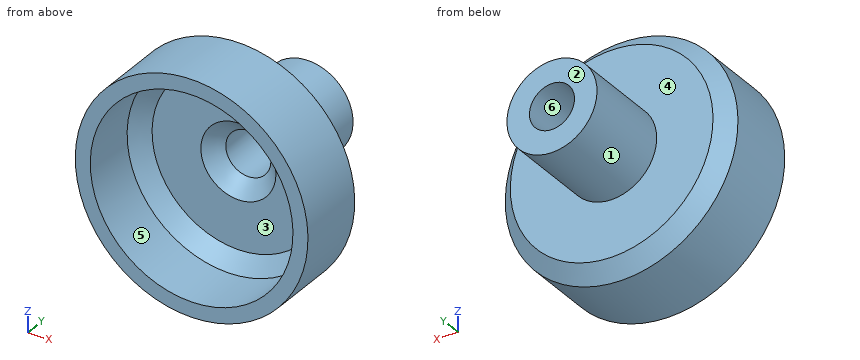
```python
from build123d import *

# Parameters (mm, degrees)
CHAMFER1_SIZE = 2
CHAMFER2_SIZE = 2


with BuildPart() as part:
    # Sketch1 → Revolve1 (revolve)
    with BuildSketch(Plane.XY, mode=Mode.PRIVATE) as revolve1_sk:
        Polygon((-15.5, 0), (-15.5, 11.4), (-6, 11.4), (-6, 23.4), (-3, 23.4), (-3, 9.4), (-13.5, 9.4), (-13.5, 0), align=None)
    revolve(revolve1_sk.sketch.rotate(Axis((0, 0, 0), (0, 1, 0)), 270), axis=Axis((0, 0, 0), (0, 1, 0)))

    # Chamfer1
    chamfer1_edges = [part.edges().sort_by_distance(p)[0] for p in [
        (0, 9.4, 13.5),
        (0, 11.4, 15.5),
    ]]
    chamfer(chamfer1_edges, length=CHAMFER1_SIZE)

    # Chamfer2
    chamfer2_edges = [part.edges().sort_by_distance(p)[0] for p in [
        (0, 9.4, 3),
    ]]
    chamfer(chamfer2_edges, length=CHAMFER2_SIZE)


solid = part.part
```
For this review, take the finished solid that the model builds, in its own axes (mm). Face numbers are marked on the shaded views. A direction names the side the tool comes from. Round coordinates to 2 decimals unless told otherwise and drop trailing zeros. Write each loop counter-clockwise with the first axis right and the second up, starting at its lowest first coordinate (ties: lowest second). Pieces come first, ordered by that corner, then holes.
1) Insertion check: pin 1 Ø1 at (x, y) = (4.5, 20) entering from +Z; pin 2 Ø1 at (y, z) = (6, 0.5) entering from -X; pin 3 Ø10 at (y, z) = (6.5, 8.5) entering from -X; pin 4 Ø1 at (x, z) = (-10, -7.5) entering from -Y. Each pin has a flat end and moves straight along its axis. Give the tip position at first contact, or say it passes through.
Answer below:
pin 1: stops at z = 4.47
pin 2: stops at x = -15.5
pin 3: stops at x = -15.1
pin 4: stops at y = 7.9
2) Take a section at A-A on x = 0. Give the boundary of the cut face in (y, z), then the cut area to 3 significant figures.
Answer below:
outline: (0, -15.5) - (9.4, -15.5) - (11.4, -13.5) - (11.4, -6) - (23.4, -6) - (23.4, -3) - (11.4, -3) - (9.4, -5) - (9.4, -11.5) - (7.4, -13.5) - (0, -13.5) - close; (0, 13.5) - (7.4, 13.5) - (9.4, 11.5) - (9.4, 5) - (11.4, 3) - (23.4, 3) - (23.4, 6) - (11.4, 6) - (11.4, 13.5) - (9.4, 15.5) - (0, 15.5) - close
area: 156 mm2
3) Mouldability with a two-part tool opening along Z and no side actions: class the marked faces 1, 2 and 3 as +Z half, -Z half, draft (parallel to the pull), parting line (faces both ways), or undercut.
Answer below:
face 1: parting line
face 2: draft
face 3: undercut
4) For line 1 along X through (y, z) = (14.5, 0); line 2 along X through (y, z) = (5.25, 0); line 3 along Y through (x, z) = (8.5, -6.5), list the stretches that pass through material, from the lowest coordinate up.
Answer below:
line 1: x = -6 to -3, 3 to 6
line 2: x = -15.5 to -13.5, 13.5 to 15.5
line 3: y = 9.4 to 11.4
5) Take a section at C-C on y = 15.5. Give the boundary of the cut face in (x, z).
Answer below:
outline: circle Ø12 at (0, 0); hole circle Ø6 at (0, 0)
6) Take a section at B-B on z = 0. Give the boundary of the cut face in (x, y).
Answer below:
outline: (-15.5, 0) - (-13.5, 0) - (-13.5, 7.4) - (-11.5, 9.4) - (-5, 9.4) - (-3, 11.4) - (-3, 23.4) - (-6, 23.4) - (-6, 11.4) - (-13.5, 11.4) - (-15.5, 9.4) - close; (3, 11.4) - (5, 9.4) - (11.5, 9.4) - (13.5, 7.4) - (13.5, 0) - (15.5, 0) - (15.5, 9.4) - (13.5, 11.4) - (6, 11.4) - (6, 23.4) - (3, 23.4) - close
7) Take a section at D-D on y = 6.75. Give the boundary of the cut face in (x, z).
Answer below:
outline: circle Ø31 at (0, 0); hole circle Ø27 at (0, 0)
8) Machinability: for the marked faces 4, 5 and 6, which of the approach directions +Z, -Z, +X, -X, +Y, -Y give a long, thin tool a straight path to every point of the face, cutting with its end or side? Answer none if there is none.
Answer below:
face 4: +Y
face 5: -Y
face 6: +Y, -Y
